from build123d import *

# Parameters (mm, degrees)
SKETCH_1_R          = 20
SKETCH_1_W          = 12.5
SKETCH_1_H          = 29.2
EXTRUDE_1_DEPTH     = 17
SKETCH_1_4_R        = 103
SKETCH_1_4_R_2      = 100
EXTRUDE_2_DEPTH     = 40
SKETCH_3_R          = 103
EXTRUDE_4_DEPTH     = 2
CUT_EXTRUDE_START   = -2
CUT_EXTRUDE_2_DEPTH = 2


# Read off the part's stored shape, not the designer's step: the extrude step
with BuildPart() as part:
    # Sketch 1 → Extrude 1 (new body)
    with BuildSketch(Plane(origin=(0, 0, 0), x_dir=(1, 0, 0), z_dir=(0, 1, 0))):
        with Locations(Location((6.25, 17.2, 0), (0, 0, 270))):
            Circle(SKETCH_1_R)
        with Locations((6.25, 14.6)):
            Rectangle(SKETCH_1_W, SKETCH_1_H, mode=Mode.SUBTRACT)
    extrude(amount=EXTRUDE_1_DEPTH)



with BuildPart() as body_2:
    # Sketch 1_4 → Extrude 2 (new body)
    with BuildSketch(Plane(origin=(0, 0, 0), x_dir=(1, 0, 0), z_dir=(0, 1, 0))):
        with Locations(Location((6.25, 17.2, 0), (0, 0, 270))):
            Circle(SKETCH_1_4_R)
        with Locations(Location((6.25, 17.2, 0), (0, 0, 270))):
            Circle(SKETCH_1_4_R_2, mode=Mode.SUBTRACT)
    extrude(amount=EXTRUDE_2_DEPTH)


with BuildPart() as part_1:
    add(part.part)

    add(body_2.part)  # Extrude 4 merges body 2
    # Sketch 3 → Extrude 4 (add)
    with BuildSketch(Plane.XZ):
        with Locations(Location((6.25, -17.2, 0), (0, 0, 90))):
            Circle(SKETCH_3_R)
    extrude(amount=EXTRUDE_4_DEPTH)

    # Cut-Extrude 2 outline → Cut-Extrude 2 (cut)
    with BuildSketch(Plane(origin=(0, 0, 0), x_dir=(1, 0, 0), z_dir=(0, 1, 0)).offset(CUT_EXTRUDE_START)):
        with BuildLine():
            Line((92.852540378, -32.8), (23.570508076, 7.2))
            ThreePointArc((23.570508076, 7.2), (16.25, -0.120508076), (6.25, -2.8))
            Line((6.25, -2.8), (6.25, -82.8))
            ThreePointArc((6.25, -82.8), (56.25, -69.402540378), (92.852540378, -32.8))
        make_face()
    extrude(amount=CUT_EXTRUDE_2_DEPTH, mode=Mode.SUBTRACT)


solid = part_1.part
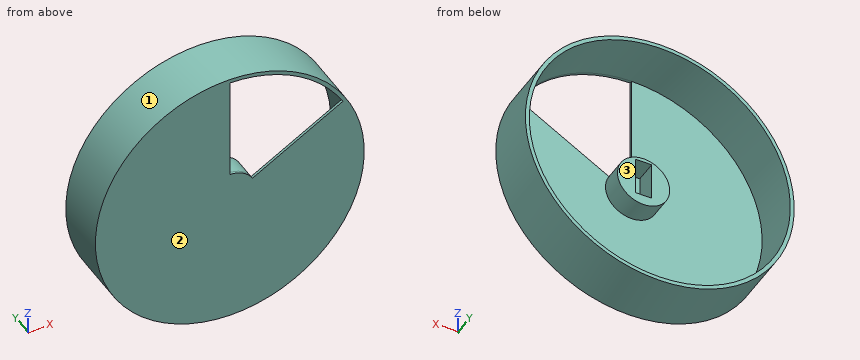
Verification items for the finished model (mm, model axes). Face numbers are marked on the shaded views. Give positions to 0.01 mm unless a question says otherwise; leave off trailing zeros. Loops run counter-clockwise (first coordinate to the right, second up) from the corner with the lowest first, then second, coordinate; pieces in that order, holes last. Notation, with made-up numbers: (45, -7.75) - (63, -7.75) arc R26 ccw to (63, 26.25) - close; hole circle Ø3 at (44, 85). An arc over 180 degrees is marked (long way). Write each question's results on one line, items separated by ' | '.
1) Mould release check, pull along Z, two halves, no side actions. Record for the marked faces 1, 2 and 3: pulls with the +Z half, pulls with the -Z half, needs draft (parallel to the pull), parting line crosses it, or undercut.
Solution:
face 1: parting line crosses it | face 2: needs draft | face 3: undercut
2) Material ranges on L1, parallel to X at y = 12.5, z = -17.2; L2, parallel to Z at x = 6, y = 23; L3, parallel to Z at x = 6, y = 14, recorded low to high. Write a range as from..to.
Solution:
L1: -96.75..-93.75, -13.75..0, 12.5..26.25, 106.25..109.25 | L2: -120.2..-117.2, 82.8..85.8 | L3: -120.2..-117.2, -37.2..-29.2, 0..2.8, 82.8..85.8
3) Sectioned sample at C-C on x = -5.5. Record the boundary of the cut face in (y, z).
Solution:
outline: (-2, -119.53) - (40, -119.53) - (40, -116.51) - (0, -116.51) - (0, -33.38) - (17, -33.38) - (17, -1.02) - (0, -1.02) - (0, 82.11) - (40, 82.11) - (40, 85.13) - (-2, 85.13) - close
4) Sectioned sample at B-B on z = 30. Record the boundary of the cut face in (x, y).
Solution:
outline: (-85.3, -2) - (6.25, -2) - (6.25, 0) - (-81.91, 0) - (-81.91, 40) - (-85.3, 40) - close; (88, -2) - (97.8, -2) - (97.8, 40) - (94.41, 40) - (94.41, 0) - (88, 0) - close
5) Sectioned sample at A-A on y = 5. Record the boundary of the cut face in (x, z), plus the area to 3 significant figures.
Solution:
outline: circle Ø206 at (6.25, -17.2); circle Ø40 at (6.25, -17.2); hole circle Ø200 at (6.25, -17.2); hole (0, -29.2) - (12.5, -29.2) - (12.5, 0) - (0, 0) - close | area: 2,800 mm2
6) Depth check by flat-ended pin: P1, Ø5, axis at y = 7, z = -10, coming from the -X side; P2, Ø2, axis at y = 25.5, z = -69.5, coming from the +X side; P3, Ø3, axis at x = -40.5, z = 15, coming from the +Y side. Enter the tip coordinate at first touch or a pass-through.
Solution:
P1: x = -96.64 | P2: x = 95.57 | P3: y = 0
7) Sectioned sample at D-D on z = -17.2. Record the boundary of the cut face in (x, y), plus the area to 3 significant figures.
Solution:
outline: (-96.75, -2) - (109.25, -2) - (109.25, 40) - (106.25, 40) - (106.25, 0) - (26.25, 0) - (26.25, 17) - (12.5, 17) - (12.5, 0) - (0, 0) - (0, 17) - (-13.75, 17) - (-13.75, 0) - (-93.75, 0) - (-93.75, 40) - (-96.75, 40) - close | area: 1,120 mm2
